from build123d import *

# Parameters (mm, degrees)
F1_DEPTH = 40
F2_DEPTH = 15
F3_SIZE  = 1


with BuildPart() as f1:
    # F0 (on Top) → F1 (new body)
    with BuildSketch(Plane.XY):
        with BuildLine():
            Line((4, 7.5), (-4, 7.5))
            ThreePointArc((-4, 7.5), (-7.5355339059, 6.0355339059), (-9, 2.5))
            Line((-9, 2.5), (-9, 0.5))
            ThreePointArc((-9, 0.5), (-6.6568542495, -5.1568542495), (-1, -7.5))
            Line((-1, -7.5), (1, -7.5))
            ThreePointArc((1, -7.5), (6.6568542495, -5.1568542495), (9, 0.5))
            Line((9, 0.5), (9, 2.5))
            ThreePointArc((9, 2.5), (7.5355339059, 6.0355339059), (4, 7.5))
        make_face()
        with BuildLine():
            ThreePointArc((-4.4, 0.9), (-3.8142135624, 2.3142135624), (-2.4, 2.9))
            Line((-2.4, 2.9), (2.4, 2.9))
            ThreePointArc((2.4, 2.9), (3.8142135624, 2.3142135624), (4.4, 0.9))
            Line((4.4, 0.9), (4.4, -0.9))
            ThreePointArc((4.4, -0.9), (3.8142135624, -2.3142135624), (2.4, -2.9))
            Line((2.4, -2.9), (-2.4, -2.9))
            ThreePointArc((-2.4, -2.9), (-3.8142135624, -2.3142135624), (-4.4, -0.9))
            Line((-4.4, -0.9), (-4.4, 0.9))
        make_face(mode=Mode.SUBTRACT)
        with BuildLine():
            Line((2.4, 2.9), (-2.4, 2.9))
            ThreePointArc((-2.4, 2.9), (-3.8142135624, 2.3142135624), (-4.4, 0.9))
            Line((-4.4, 0.9), (-4.4, -0.9))
            ThreePointArc((-4.4, -0.9), (-3.8142135624, -2.3142135624), (-2.4, -2.9))
            Line((-2.4, -2.9), (2.4, -2.9))
            ThreePointArc((2.4, -2.9), (3.8142135624, -2.3142135624), (4.4, -0.9))
            Line((4.4, -0.9), (4.4, 0.9))
            ThreePointArc((4.4, 0.9), (3.8142135624, 2.3142135624), (2.4, 2.9))
        make_face()
    extrude(amount=-F1_DEPTH)

    # F0 (on Top) → F2 (join)
    with BuildSketch(Plane.XY):
        with BuildLine():
            Line((2.4, 2.9), (-2.4, 2.9))
            ThreePointArc((-2.4, 2.9), (-3.8142135624, 2.3142135624), (-4.4, 0.9))
            Line((-4.4, 0.9), (-4.4, -0.9))
            ThreePointArc((-4.4, -0.9), (-3.8142135624, -2.3142135624), (-2.4, -2.9))
            Line((-2.4, -2.9), (2.4, -2.9))
            ThreePointArc((2.4, -2.9), (3.8142135624, -2.3142135624), (4.4, -0.9))
            Line((4.4, -0.9), (4.4, 0.9))
            ThreePointArc((4.4, 0.9), (3.8142135624, 2.3142135624), (2.4, 2.9))
        make_face()
    extrude(amount=F2_DEPTH)

    # F3
    f3_edges = [f1.edges().sort_by_distance(p)[0] for p in [
        (0, 2.9, 15),
        (-3.814214, 2.314214, 15),
        (-4.4, 0, 15),
        (-3.814214, -2.314214, 15),
        (0, -2.9, 15),
        (3.814214, -2.314214, 15),
        (4.4, 0, 15),
        (3.814214, 2.314214, 15),
    ]]
    chamfer(f3_edges, length=F3_SIZE)


solid = f1.part
Could you check a few things on this model? Use its own coordinates, in mm. A direction names the side the tool comes from. Coordinates: 2 decimals unless noted, no trailing zeros. Write each loop counter-clockwise with the first axis right and the second up, starting at its lowest first coordinate (ties: lowest second). Pieces come first, ordered by that corner, then holes. Notation, with made-up numbers: M 61,-13.75 L 103,-13.75 A21 cw 103,15.25 Z; hole C 27.25,50.5 d10. An arc over 180 degrees is marked long. One line per question, with ' | ' between items.
1) I need wall thicknesses on probe 1 along Z at (x, y) = (3, 3.25); probe 2 along Y at (x, z) = (2, 5.5); probe 3 along X at (y, z) = (0.25, -35). Which ranges of each line are inside material? Lowest first, please. Write a range as [from, to].
Checks:
probe 1: [-40, 0] | probe 2: [-2.9, 2.9] | probe 3: [-9, 9]
2) Imagine slicing it at B-B, the plane x = -0.5. Write out the boundary of the cut face in (y, z), and give its area (3 significant figures).
Checks:
outline: M -7.5,-40 L 7.5,-40 L 7.5,0 L 2.9,0 L 2.9,14 L 1.9,15 L -1.9,15 L -2.9,14 L -2.9,0 L -7.5,0 Z | area: 686 mm²
3) For pin 1 Ø1.5 at (y, z) = (4.5, -7) entering from -X; pin 2 Ø4 at (y, z) = (-3, -19.5) entering from +X; pin 3 Ø0.9 at (y, z) = (0, 7.5) entering from +X, each with a flat end and sliding along its axis, tell me the tip position at first contact or that it passes through.
Checks:
pin 1: x = -8.84 | pin 2: x = 8.86 | pin 3: x = 4.4
4) Imagine slicing it at C-C, the plane y = 3.5. Write out the boundary of the cut face in (x, z).
Checks:
outline: M -8.9,-40 L 8.9,-40 L 8.9,0 L -8.9,0 Z
5) Imagine slicing it at A-A, the plane z = -23.5. Write out the boundary of the cut face in (x, y).
Checks:
outline: M -9,0.5 A8 ccw -1,-7.5 L 1,-7.5 A8 ccw 9,0.5 L 9,2.5 A5 ccw 4,7.5 L -4,7.5 A5 ccw -9,2.5 Z
6) For faces 1 (the face through (-3.83, -2.3, 6.9)), 2 (the face through (-4.4, 0, 7)), 3 (the face through (0, -2.9, 7)), 4 (the face through (6.594, -5.219, -19.72)), 5 (the face through (4.4, 0, 7)), which set-ups out of +Z, -Z, +X, -X, +Y, -Y let a thin tool reach every point of the face, with its end or its side?
Checks:
face 1: +Z, -X, -Y | face 2: +Z, -X, +Y, -Y | face 3: +Z, +X, -X, -Y | face 4: +Z, -Z, +X, -Y | face 5: +Z, +X, +Y, -Y
7) Imagine slicing it at D-D, the plane x = 7. Write out the boundary of the cut face in (y, z).
Checks:
outline: M -4.79,-40 L 6.5,-40 L 6.5,0 L -4.79,0 Z
